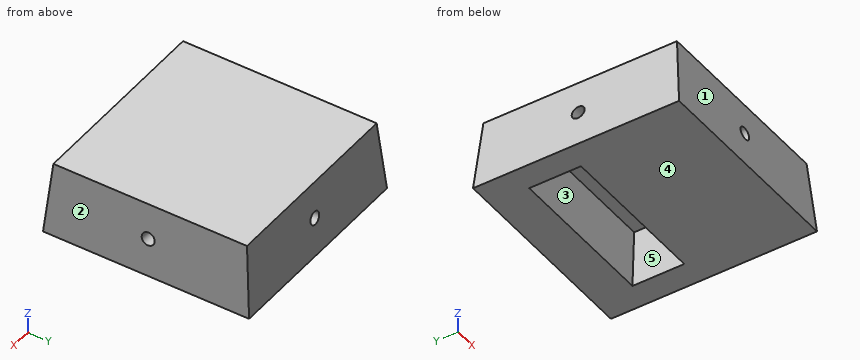
from build123d import *

# Parameters (mm, degrees)
F0_W        = 101.6
F0_H        = 101.6
F1_DEPTH    = 34.925
F2_T1_DEPTH = 299.3404177556
F2_T3_DEPTH = 299.3404177556
F3_R        = 3.175
F4_DEPTH    = 12.7
F5_R        = 3.175
F6_DEPTH    = 12.7
F7_R        = 3.175
F8_DEPTH    = 12.7
F9_R        = 3.175
F10_DEPTH   = 12.7
F11_W       = 75.6562831473
F11_H       = 25.4
F12_DEPTH   = 25.4
F13_SIZE2   = 2.53999
F13_SIZE    = 25.39999


# Not quite as in the source:
# - a fillet or chamfer that OpenCascade refuses, or shapes differently, is made with other operations: its cross-section is extruded or revolved along the edge and cut away or added
# - a fillet or chamfer is up to 0.001 mm smaller than in the source, because OpenCascade refuses the exact size


with BuildPart() as f1:
    # F0 (on Top) → F1 (new body)
    with BuildSketch(Plane.XY):
        Rectangle(F0_W, F0_H)
    extrude(amount=F1_DEPTH)

    # F2: chamfer of 3.3274 x 38.0323560322 on 4 edges, made by hand

    # F2_s2 → F2_t1 (cut)
    with BuildSketch(Plane.XZ.offset(-149.6702088778)):
        Polygon((-50.8, -3.1073560322), (-47.4726, 34.925), (-50.8, 34.925), align=None)
        Polygon((50.8, -3.1073560322), (47.4726, 34.925), (50.8, 34.925), align=None)
    extrude(amount=F2_T1_DEPTH, mode=Mode.SUBTRACT)

    # F2_s4 → F2_t3 (cut)
    with BuildSketch(Plane.YZ.offset(-149.6702088778)):
        Polygon((-50.8, -3.1073560322), (-47.4726, 34.925), (-50.8, 34.925), align=None)
        Polygon((50.8, -3.1073560322), (47.4726, 34.925), (50.8, 34.925), align=None)
    extrude(amount=F2_T3_DEPTH, mode=Mode.SUBTRACT)

    # F3 (on face) → F4 (cut)
    with BuildSketch(Plane(origin=(0, 50.1443235703, 4.3870598526), x_dir=(-1, 0, 0), z_dir=(0, 0.9961946981, 0.0871557427))):
        with Locations((0, 13.6719250414)):
            Circle(F3_R)
    extrude(amount=-F4_DEPTH, mode=Mode.SUBTRACT)

    # F5 (on face) → F6 (cut)
    with BuildSketch(Plane(origin=(0, -50.1443235703, 4.3870598526), x_dir=(1, 0, 0), z_dir=(0, -0.9961946981, 0.0871557427))):
        with Locations((0, 13.6719250414)):
            Circle(F5_R)
    extrude(amount=-F6_DEPTH, mode=Mode.SUBTRACT)

    # F7 (on face) → F8 (cut)
    with BuildSketch(Plane(origin=(50.1443235703, 0, 4.3870598526), x_dir=(0, 1, 0), z_dir=(0.9961946981, 0, 0.0871557427))):
        with Locations((0, 13.6719250414)):
            Circle(F7_R)
    extrude(amount=-F8_DEPTH, mode=Mode.SUBTRACT)

    # F9 (on face) → F10 (cut)
    with BuildSketch(Plane(origin=(-50.1443235703, 0, 4.3870598526), x_dir=(0, -1, 0), z_dir=(-0.9961946981, 0, 0.0871557427))):
        with Locations((0, 13.6719250414)):
            Circle(F9_R)
    extrude(amount=-F10_DEPTH, mode=Mode.SUBTRACT)

    # F11 (on face) → F12 (cut)
    with BuildSketch(Plane(origin=(0, 0, 0), x_dir=(1, 0, 0), z_dir=(0, 0, -1))):
        with Locations((0, -18.7781415736)):
            Rectangle(F11_W, F11_H)
    extrude(amount=-F12_DEPTH, mode=Mode.SUBTRACT)

    # F13 (size 25.4 and 2.54 in the source; OpenCascade refuses exactly that, so slightly less here)
    f13_edges = [f1.edges().sort_by_distance(p)[0] for p in [
        (0, 6.078142, 25.4),
        (-37.828142, 18.778142, 25.4),
        (37.828142, 18.778142, 25.4),
        (0, 31.478142, 25.4),
    ]]
    chamfer(f13_edges, length=F13_SIZE, length2=F13_SIZE2)


solid = f1.part
Read the model definition and answer for the solid it produces. Units are mm, in the model's axes. Face numbers are marked on the shaded views. A direction names the side the tool comes from. Round coordinates to 2 decimals unless told otherwise and drop trailing zeros. Write each loop counter-clockwise with the first axis right and the second up, starting at its lowest first coordinate (ties: lowest second). Pieces come first, ordered by that corner, then holes.
1. The part is cut by section D-D, the plane z = 5. Determine the outline of the cut face in (x, y).
2. The part is cut by section A-A, the plane z = 24. Determine the outline of the cut face in (x, y).
3. Given pin 1 Ø1.5 at (y, z) = (-7, 31.5) entering from -X; pin 2 Ø5 at (x, y) = (-32, -25) entering from -Z; pin 3 Ø10 at (x, y) = (-8, 17.5) entering from -Z; pin 4 Ø4 at (y, z) = (17, 31) entering from +X, each flat-ended and moving along its own axis, determine where each tip first touches the part or whether it passes through.
4. Determine the mould class of the marked faces 1, 2 and 3 for opening direction Y: pulls with the +Y half, pulls with the -Y half, needs draft (parallel to the pull), parting line crosses it, or undercut.
5. Straight lines are drawn through the part: L1, parallel to X at y = 10, z = 5; L2, parallel to Y at x = 41, z = 18.5; L3, parallel to Y at x = 11, z = 25. For each, find the intervals that lie inside material, in ascending order.
6. Which of the six approach directions +Z, -Z, +X, -X, +Y, -Y give full straight-line access (tool end or side, diameter ignored) to the marked faces 4 and 5?
Values:
1. outline: (-50.09, -50.09) - (50.09, -50.09) - (50.09, 50.09) - (-50.09, 50.09) - close; hole (-37.33, 6.58) - (37.33, 6.58) - (37.33, 30.98) - (-37.33, 30.98) - close
2. outline: (-48.43, -48.43) - (48.43, -48.43) - (48.43, 48.43) - (-48.43, 48.43) - close; hole (-35.43, 8.48) - (35.43, 8.48) - (35.43, 29.08) - (-35.43, 29.08) - close
3. pin 1: stops at x = -47.84
3. pin 2: stops at z = 0
3. pin 3: stops at z = 25.4
3. pin 4: stops at x = 47.99
4. face 1: pulls with the -Y half
4. face 2: needs draft
4. face 3: undercut
5. L1: x = -50.09 to -37.33, 37.33 to 50.09
5. L2: y = -48.91 to -2.95, 2.95 to 48.91
5. L3: y = -48.34 to 8.58, 28.98 to 48.34
6. face 4: -Z, +X, -X, +Y, -Y
6. face 5: -Z
